Input: part model. Units: mm. Frame: model coordinates. Face numbers are marked on the shaded views. A direction names the side the tool comes from. Coordinates: 2 decimals unless noted, no trailing zeros. Loops run counter-clockwise (first coordinate to the right, second up) from the corner with the lowest first, then second, coordinate; pieces in that order, holes last. Notation, with made-up numbers: M 66,49.25 L 119,49.25 A23 cw 119,59.25 Z; hole C 39,44 d5. An arc over 180 degrees is marked long. Use a Markdown table: item, result. Add a question column.
1. Section C-C on z = 45. Output: boundary loops of the cut face in (x, y).
2. Section B-B on y = 15. Output: boundary loops of the cut face in (x, z).
3. Set-up query: the marked faces 1 and 2. Return all of +Z, -Z, +X, -X, +Y, -Y with unobstructed straight access to the full face (end or side cutting, diameter ignored); none if empty.
4. Pin query (flat end, axial travel): pin 1 (2 mm diameter, centred on x = 11.5, z = 42, fed in from +Y); pin 2 (5 mm diameter, centred on x = 59.5, y = 10.5, fed in from +Z). Return the tip coordinate at first contact, or that it passes through.
5. Section D-D on x = 4. Output: boundary loops of the cut face in (y, z).
6. Section A-A on x = 14. Output: boundary loops of the cut face in (y, z).
7. Line query: L1, parallel to X at y = 0.6, z = 4.5; L2, parallel to Z at x = 32, y = 9. Output: solid intervals per line, ascending. Write a range as [from, to].
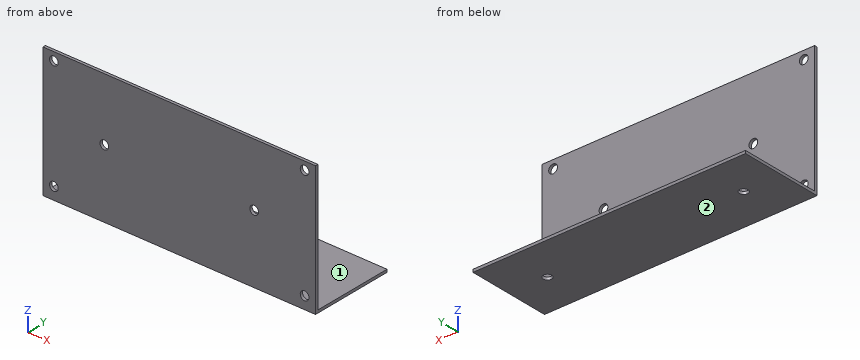
```python
from build123d import *

# Parameters (mm, degrees)
EXTRUDE_1_DEPTH     = 100
SKETCH_2_R          = 1.6
CUT_EXTRUDE_1_DEPTH = 1
SKETCH_3_R          = 1.6
CUT_EXTRUDE_2_DEPTH = 1
SKETCH1_R           = 1.6
CUT_EXTRUDE1_DEPTH  = 10


with BuildPart() as part:
    # Эскиз1 → Бобышка-Вытянуть1 (new body)
    with BuildSketch(Plane(origin=(0, 0, 0), x_dir=(0, 0, -1), z_dir=(1, 0, 0))):
        Polygon((0, 0), (-48, 0), (-48, 1), (-1, 1), (-1, 30.5), (0, 30.5), align=None)
    extrude(amount=EXTRUDE_1_DEPTH)

    # Эскиз2 → Вырез-Вытянуть1 (cut)
    with BuildSketch(Plane(origin=(0, 0, 0), x_dir=(-1, 0, 0), z_dir=(0, 0, -1))):
        with Locations((-86, 15)):
            Circle(SKETCH_2_R)
        with Locations((-14, 15)):
            Circle(SKETCH_2_R)
    extrude(amount=-CUT_EXTRUDE_1_DEPTH, mode=Mode.SUBTRACT)

    # Эскиз3 → Вырез-Вытянуть2 (cut)
    with BuildSketch(Plane.XZ):
        with Locations(Location((22.5, 25, 0), (0, 0, 270))):
            Circle(SKETCH_3_R)
        with Locations(Location((77.5, 25, 0), (0, 0, 270))):
            Circle(SKETCH_3_R)
    extrude(amount=-CUT_EXTRUDE_2_DEPTH, mode=Mode.SUBTRACT)

    # Sketch1 → Cut-Extrude1 (cut)
    with BuildSketch(Plane.XZ):
        with Locations(Location((4, 45, 0), (0, 0, 270))):
            Circle(SKETCH1_R)
        with Locations(Location((96, 45, 0), (0, 0, 270))):
            Circle(SKETCH1_R)
        with Locations(Location((96, 4.5, 0), (0, 0, 270))):
            Circle(SKETCH1_R)
        with Locations(Location((4, 4.5, 0), (0, 0, 270))):
            Circle(SKETCH1_R)
    extrude(amount=-CUT_EXTRUDE1_DEPTH, mode=Mode.SUBTRACT)


solid = part.part
```
Answers below:
| question | item | result |
|---|---|---|
| 1 | outline | M 0,0 L 2.4,0 L 2.4,1 L 0,1 Z; M 5.6,0 L 94.4,0 L 94.4,1 L 5.6,1 Z; M 97.6,0 L 100,0 L 100,1 L 97.6,1 Z |
| 2 | outline | M 0,0 L 12.4,0 L 12.4,1 L 0,1 Z; M 15.6,0 L 84.4,0 L 84.4,1 L 15.6,1 Z; M 87.6,0 L 100,0 L 100,1 L 87.6,1 Z |
| 3 | face 1 | +Z, +X, -X, +Y |
| 3 | face 2 | -Z, +X, -X, +Y, -Y |
| 4 | pin 1 | stops at y = 1 |
| 4 | pin 2 | stops at z = 1 |
| 5 | outline | M 0,0 L 30.5,0 L 30.5,1 L 1,1 L 1,2.9 L 0,2.9 Z; M 0,6.1 L 1,6.1 L 1,43.4 L 0,43.4 Z; M 0,46.6 L 1,46.6 L 1,48 L 0,48 Z |
| 6 | outline | M 0,0 L 13.4,0 L 13.4,1 L 1,1 L 1,48 L 0,48 Z; M 16.6,0 L 30.5,0 L 30.5,1 L 16.6,1 Z |
| 7 | L1 | x = [0, 2.4], [5.6, 94.4], [97.6, 100] |
| 7 | L2 | z = [0, 1] |
